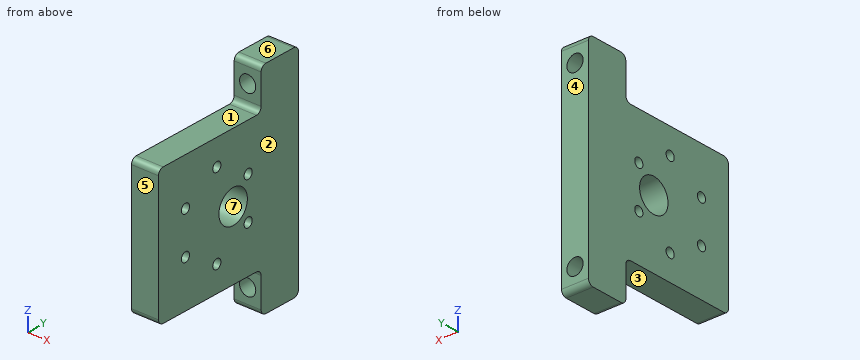
from build123d import *

# Parameters (mm, degrees)
SKETCH1_W           = 80
SKETCH1_H           = 60
BOSS_EXTRUDE1_DEPTH = 10
SKETCH2_R           = 6.1
CUT_EXTRUDE1_DEPTH  = 55.083269132
SKETCH3_R           = 1.75
CUT_EXTRUDE3_DEPTH  = 55.083269132
SKETCH4_W           = 15
SKETCH4_H           = 44
CUT_EXTRUDE4_DEPTH  = 50
SKETCH5_R           = 3
CUT_EXTRUDE5_DEPTH  = 50
FILLET1_R           = 2


with BuildPart() as part:
    # Sketch1 → Boss-Extrude1 (new body)
    with BuildSketch(Plane(origin=(0, 0, 0), x_dir=(0, 0, -1), z_dir=(1, 0, 0))):
        with Locations((0, 5)):
            Rectangle(SKETCH1_W, SKETCH1_H)
    extrude(amount=BOSS_EXTRUDE1_DEPTH)

    # Sketch2 → Cut-Extrude1 (cut, through all)
    with BuildSketch(Plane(origin=(10, 0, 0), x_dir=(0, 0, -1), z_dir=(1, 0, 0))):
        with Locations(Location((0, 7, 0), (0, 0, 180))):
            Circle(SKETCH2_R)
    extrude(amount=-CUT_EXTRUDE1_DEPTH, mode=Mode.SUBTRACT)

    # Sketch3 → Cut-Extrude3 (cut, through all)
    with BuildSketch(Plane(origin=(10, 0, 0), x_dir=(0, 0, -1), z_dir=(1, 0, 0))):
        with Locations((7.75, -13.423393759)):
            Circle(SKETCH3_R)
        with Locations(Location((-7.75, -13.423393759, 0), (0, 0, 180))):
            Circle(SKETCH3_R)
        with Locations((-7.75, 13.423393759)):
            Circle(SKETCH3_R)
        with Locations(Location((7.75, 13.423393759, 0), (0, 0, 180))):
            Circle(SKETCH3_R)
        with Locations((15.5, 0)):
            Circle(SKETCH3_R)
        with Locations(Location((-15.5, 0, 0), (0, 0, 180))):
            Circle(SKETCH3_R)
    extrude(amount=-CUT_EXTRUDE3_DEPTH, mode=Mode.SUBTRACT)

    # Sketch4 → Cut-Extrude4 (cut)
    with BuildSketch(Plane(origin=(10, 0, 0), x_dir=(0, 0, -1), z_dir=(1, 0, 0))):
        with Locations((-32.5, -3)):
            Rectangle(SKETCH4_W, SKETCH4_H)
        with Locations((32.5, -3)):
            Rectangle(SKETCH4_W, SKETCH4_H)
    extrude(amount=-CUT_EXTRUDE4_DEPTH, mode=Mode.SUBTRACT)

    # Sketch5 → Cut-Extrude5 (cut)
    with BuildSketch(Plane(origin=(0, 35, 0), x_dir=(1, 0, 0), z_dir=(0, 1, 0))):
        with Locations(Location((5, 32.5, 0), (0, 0, 270))):
            Circle(SKETCH5_R)
        with Locations(Location((5, -32.5, 0), (0, 0, 270))):
            Circle(SKETCH5_R)
    extrude(amount=-CUT_EXTRUDE5_DEPTH, mode=Mode.SUBTRACT)

    # Fillet1
    fillet1_edges = [part.edges().sort_by_distance(p)[0] for p in [
        (5, 19, 40),
        (5, 19, 25),
        (5, -25, 25),
        (5, -25, -25),
        (5, 19, -25),
        (5, 19, -40),
        (5, 35, 40),
        (5, 35, -40),
    ]]
    fillet(fillet1_edges, radius=FILLET1_R)


solid = part.part
CAD build for the part. Positions are in the model's coordinates, mm. Face numbers are marked on the shaded views. A direction names the side the tool comes from. Round coordinates to 2 decimals unless told otherwise and drop trailing zeros. Order: outer loops, then holes, each group sorted by start corner. A loop starts at its lowest first (then second) coordinate and runs counter-clockwise, first axis right, second up. Notation, with made-up numbers: (59.5, 40.25) -> (89.5, 40.25) arc R32 cw to (89.5, 79.25) -> close; hole circle Ø2 at (72.25, 65.25). An arc over 180 degrees is marked (long way). Write item = value, one per line. Start each with the question number.
(1) Cut at D-D, the plane z = -31.5. List the corners of the cut face in (x, y), then the cut area to 3 significant figures.
(2) Pull direction Y, two halves, no side cores. Call the marked faces 4, 5, 6 and 7: released by +Y, released by -Y, zero draft, split by the parting line, or undercut.
(3) Cut at A-A, the plane y = 7. List the corners of the cut face in (x, z).
(4) Probe line 1 (Y direction, x = 7.25, z = 7.75); line 2 (Y direction, x = 8, z = 0); line 3 (Y direction, x = 2.75, z = -15.5). List the from-to ranges inside material, lowest first. Write a range as [from, to].
(5) Cut at C-C, the plane x = 7. State how many separate pieces and enclosed holes the cut face has, then the cut area to 3 significant figures.
(6) Pin check, flat tips, straight feed: P1, Ø3, axis at y = -13.42, z = 7.75, coming from the +X side; P2, Ø3, axis at x = 3.5, z = -31.5, coming from the -Y side; P3, Ø3, axis at x = 5, y = -17, coming from the +Z side; P4, Ø4, axis at x = 7, y = -16, coming from the -Z side. Stop position of each tip, or through.
(7) Cut at B-B, the plane z = 7.75. List the corners of the cut face in (x, y), then the cut area to 3 significant figures.
(8) Which spindle directions (+Z, -Z, +X, -X, +Y, -Y) get a long thin tool onto all of the face, cutting with end or side? Do the marked faces 1, 2 and 3. Say none if no direction does.
Model answer:
q1.outline = (0, 19) -> (2.17, 19) -> (2.17, 35) -> (0, 35) -> close; (7.83, 19) -> (10, 19) -> (10, 35) -> (7.83, 35) -> close
q1.area = 69.5 mm2
q2.face_4 = released by +Y
q2.face_5 = released by -Y
q2.face_6 = zero draft
q2.face_7 = undercut
q3.outline = (0, -25) -> (10, -25) -> (10, -6.1) -> (0, -6.1) -> close; (0, 6.1) -> (10, 6.1) -> (10, 25) -> (0, 25) -> close
q4.line_1 = [-25, -15.17], [-11.67, 11.67], [15.17, 35]
q4.line_2 = [-25, 0.9], [13.1, 35]
q4.line_3 = [-25, -1.75], [1.75, 35]
q5.separate_pieces = 3
q5.enclosed_holes = 7
q5.area = 3,160 mm2
q6.P1 = through
q6.P2 = 19
q6.P3 = 25
q6.P4 = -25
q7.outline = (0, -25) -> (10, -25) -> (10, -15.17) -> (0, -15.17) -> close; (0, -11.67) -> (10, -11.67) -> (10, 11.67) -> (0, 11.67) -> close; (0, 15.17) -> (10, 15.17) -> (10, 35) -> (0, 35) -> close
q7.area = 530 mm2
q8.face_1 = +Z, +X, -X, -Y
q8.face_2 = +Z, -Z, +X, +Y, -Y
q8.face_3 = -Z, +X, -X, -Y
